The drawing under review shows one solid part. Ordinate dimensions are in mm from its lowest x, y, z. A direction names the side the tool comes from. Give positions to 0.01 mm unless a question says otherwise; leave off trailing zeros. Write each loop counter-clockwise with the first axis right and the second up, starting at its lowest first coordinate (ties: lowest second). Pieces come first, ordered by that corner, then holes. Notation, with made-up numbers: M 11.5,-38 L 58.5,-38 A8 cw 58.5,-28 Z; hole C 8,-32 d7. An arc over 180 degrees is marked long. Answer as a JSON object with one key per item and string values. Group by question number.
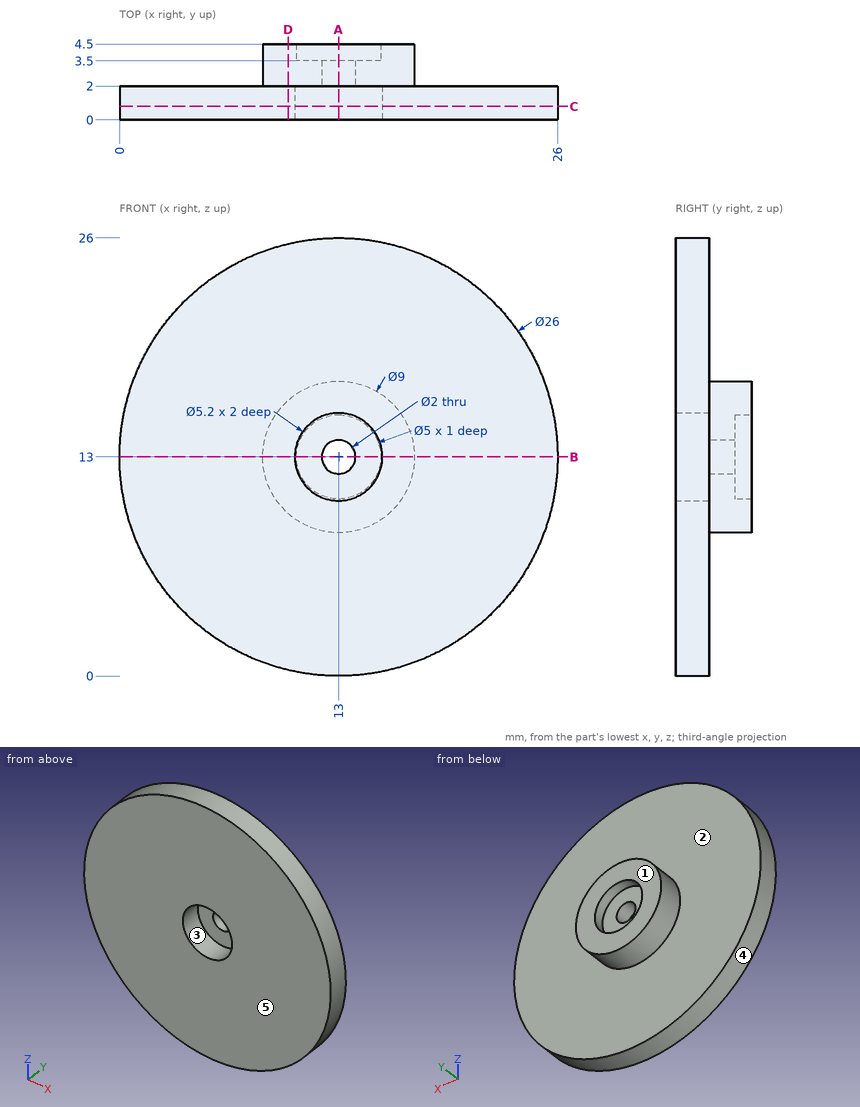
Item 1: Consider section D-D (x = 10). Give the boundary of the cut face in (y, z), plus the area to 3 significant figures.
Item 2: Consider section A-A (x = 13). Give the boundary of the cut face in (y, z).
Item 3: Consider section B-B (z = 13). Give the boundary of the cut face in (x, y).
Item 4: Machinability: for the marked faces 1 and 2, which of the approach directions +Z, -Z, +X, -X, +Y, -Y give a long, thin tool a straight path to every point of the face, cutting with its end or side? Answer none if there is none.
Item 5: Draft analysis for pull direction X (two halves, no side actions). For the marked faces 3, 4 and 5, state which applies: released by +X, released by -X, zero draft, split by the parting line, or undercut.
Item 6: Consider section C-C (y = 0.8). Give the boundary of the cut face in (x, z).
Item 7: Insertion check: P1, Ø10, axis at x = 15.5, z = 3.5, coming from the +Y side; P2, Ø2.5, axis at x = 13, z = 13, coming from the -Y side; P3, Ø1, axis at y = 3.5, z = 20, coming from the -X side. Each pin has a flat end and moves straight along its axis. Give the tip position at first contact, or say it passes through.
Item 8: To check wall thickness, follow probe 1 along X at (y, z) = (0.55, 13); probe 2 along X at (y, z) = (3.85, 13); probe 3 along Y at (x, z) = (20.75, 9.5). State the ranges of each line that lie inside material, in increasing order.
Result set:
{
 "1": {"outline": "M 0,0.35 L 2,0.35 L 2,9.65 L 4.5,9.65 L 4.5,16.35 L 2,16.35 L 2,25.65 L 0,25.65 Z", "area": "67.4 mm^2"},
 "2": {"outline": "M 0,0 L 2,0 L 2,8.5 L 4.5,8.5 L 4.5,10.5 L 3.5,10.5 L 3.5,12 L 2,12 L 2,10.4 L 0,10.4 Z; M 0,15.6 L 2,15.6 L 2,14 L 3.5,14 L 3.5,15.5 L 4.5,15.5 L 4.5,17.5 L 2,17.5 L 2,26 L 0,26 Z"},
 "3": {"outline": "M 0,0 L 10.4,0 L 10.4,2 L 12,2 L 12,3.5 L 10.5,3.5 L 10.5,4.5 L 8.5,4.5 L 8.5,2 L 0,2 Z; M 14,2 L 15.6,2 L 15.6,0 L 26,0 L 26,2 L 17.5,2 L 17.5,4.5 L 15.5,4.5 L 15.5,3.5 L 14,3.5 Z"},
 "4": {"face 1": "+Z, -Z, +X, -X, +Y", "face 2": "+Y"},
 "5": {"face 3": "undercut", "face 4": "split by the parting line", "face 5": "zero draft"},
 "6": {"outline": "C 13,13 d26; hole C 13,13 d5.2"},
 "7": {"P1": "stops at y = 2", "P2": "stops at y = 2", "P3": "passes through"},
 "8": {"probe 1": "x = 0 to 10.4, 15.6 to 26", "probe 2": "x = 8.5 to 10.5, 15.5 to 17.5", "probe 3": "y = 0 to 2"}
}
